```python
from build123d import *

# Parameters (mm, degrees)
ESTRUSIONE_ESTRUSIONE1_DEPTH = 5
SCHIZZO2_R                   = 1.625
TAGLIO_ESTRUSIONE1_DEPTH     = 11.10267083
SCHIZZO3_R                   = 2.5
TAGLIO_ESTRUSIONE2_DEPTH     = 3.5
RACCORDO1_R                  = 10
SCHIZZO4_W                   = 2.5
SCHIZZO4_H                   = 5
TAGLIO_ESTRUSIONE3_DEPTH     = 10
RACCORDO2_R                  = 1
SCHIZZO5_R                   = 1.625
TAGLIO_ESTRUSIONE4_DEPTH     = 10


with BuildPart() as part:
    # Schizzo1 → Estrusione-Estrusione1 (new body, symmetric)
    with BuildSketch(Plane(origin=(0, 0, 0), x_dir=(0, 0, -1), z_dir=(1, 0, 0))):
        Polygon((-21.188457268, 88.94490566), (-26.688457268, 88.94490566), (-26.688457268, 109.666731067), (-40, 122.978273799), (-40, 147.94490566), (-18, 169.94490566), (-16.585786438, 168.530692098), (-25, 160.116478536), (-25, 158.94490566), (-20, 158.94490566), (-34.5, 144.44490566), (-34.5, 125.256448392), (-21.188457268, 111.94490566), align=None)
    extrude(amount=ESTRUSIONE_ESTRUSIONE1_DEPTH, both=True)

    # Schizzo2 → Taglio-Estrusione1 (cut, through all)
    with BuildSketch(Plane.XY.offset(26.688457268)):
        with Locations((0, 92.723474812)):
            Circle(SCHIZZO2_R)
    extrude(amount=-TAGLIO_ESTRUSIONE1_DEPTH, mode=Mode.SUBTRACT)

    # Schizzo3 → Taglio-Estrusione2 (cut)
    with BuildSketch(Plane.XY.offset(26.688457268)):
        with Locations((0, 92.723474812)):
            Circle(SCHIZZO3_R)
    extrude(amount=-TAGLIO_ESTRUSIONE2_DEPTH, mode=Mode.SUBTRACT)

    # Raccordo1
    raccordo1_edges = [part.edges().sort_by_distance(p)[0] for p in [
        (0, 109.666731067, 26.688457268),
        (0, 122.978273799, 40),
        (0, 147.94490566, 40),
        (0, 144.44490566, 34.5),
        (0, 125.256448392, 34.5),
    ]]
    fillet(raccordo1_edges, radius=RACCORDO1_R)

    # Schizzo4 → Taglio-Estrusione3 (cut)
    with BuildSketch(Plane.ZY.offset(5)):
        with Locations((38.75, 141.44490566)):
            Rectangle(SCHIZZO4_W, SCHIZZO4_H)
    extrude(amount=-TAGLIO_ESTRUSIONE3_DEPTH, mode=Mode.SUBTRACT)

    # Raccordo2
    raccordo2_edges = [part.edges().sort_by_distance(p)[0] for p in [
        (0, 158.94490566, 25),
    ]]
    fillet(raccordo2_edges, radius=RACCORDO2_R)

    # Schizzo5 → Taglio-Estrusione4 (cut)
    with BuildSketch(Plane(origin=(0, 93.97245283, 93.97245283), x_dir=(1, 0, 0), z_dir=(0, 0.707106781, 0.707106781))):
        with Locations((0, 103.441273159)):
            Circle(SCHIZZO5_R)
    extrude(amount=-TAGLIO_ESTRUSIONE4_DEPTH, mode=Mode.SUBTRACT)


solid = part.part
```
Geometry check sheet. Reference: the model listing, model coordinates, mm. A direction names the side the tool comes from. Give positions to 0.01 mm unless a question says otherwise; leave off trailing zeros. Write each loop counter-clockwise with the first axis right and the second up, starting at its lowest first coordinate (ties: lowest second). Pieces come first, ordered by that corner, then holes.
1) Section check C-C, the plane x = 0. State how many separate pieces and enclosed holes the cut face has, and give its area (3 significant figures).
2) Section check B-B, the plane x = 4.25. Record the boundary of the cut face in (y, z).
3) Release check for a two-part mould opening along Z. For faces 4 (the flat face through (2, 93, 23.188)), 5 (the cylindrical face through (-0.07, 144.18, 33.718)), 6 (the cylindrical face through (-0.352, 165.298, 21.253)) record: pulls with the +Z half, pulls with the -Z half, needs draft (parallel to the pull), parting line crosses it, or undercut.
4) Section check A-A, the plane z = 28.5. Record the boundary of the cut face in (x, y), and give its area (3 significant figures).
5) Material ranges on L1, parallel to Y at x = 0, z = 25.85; L2, parallel to X at y = 93, z = 25.25; L3, parallel to Y at x = -1.5, z = 25.25, recorded low to high.
6) Section check D-D, the plane z = 33.5. Record the boundary of the cut face in (x, y), and give its area (3 significant figures).
7) Gauge pin test, flat ends, axial feed: pin 1 (1 mm diameter, centred on x = 2.5, y = 100.5, fed in from +Z); pin 2 (1.5 mm diameter, centred on x = -1, z = 29.5, fed in from -Y); pin 3 (3 mm diameter, centred on x = 0.5, z = 22, fed in from +Y). Record the tip position at first contact, or that the pin passes through.
8) Access from +Z, -Z, +X, -X, +Y, -Y to the whole of each face (thin tool, end or side, straight path). Record for faces 1 (the flat face through (0, 101, 21.188)), 2 (the flat face through (0, 138.945, 39)), 3 (the cylindrical face through (0.07, 125.521, 33.718)).
Computed:
1. separate pieces: 3
1. enclosed holes: 0
1. area: 449 mm2
2. outline: (88.94, 21.19) - (111.94, 21.19) - (122.33, 31.57) arc R10 cw to (129.4, 34.5) - (140.3, 34.5) arc R10 cw to (147.37, 31.57) - (158.94, 20) - (158.94, 24) arc R1 cw to (159.94, 25) - (160.12, 25) - (168.53, 16.59) - (169.94, 18) - (150.87, 37.07) arc R10 ccw to (143.94, 40) - (143.94, 37.5) - (138.94, 37.5) - (138.94, 40) - (127.12, 40) arc R10 ccw to (120.05, 37.07) - (112.6, 29.62) arc R10 cw to (105.52, 26.69) - (88.94, 26.69) - close
3. face 4: pulls with the +Z half
3. face 5: pulls with the -Z half
3. face 6: undercut
4. outline: (-5, 111.26) - (5, 111.26) - (5, 119.26) - (-5, 119.26) - close; (-5, 150.44) - (5, 150.44) - (5, 159.44) - (-5, 159.44) - close
4. area: 170 mm2
5. L1: y = 88.94 to 90.22, 95.22 to 116.61, 153.09 to 162.09
5. L2: x = -5 to -2.48, 2.48 to 5
5. L3: y = 88.94 to 90.72, 94.72 to 116.01, 153.69 to 162.69
6. outline: (-5, 116.48) - (5, 116.48) - (5, 125.04) - (-5, 125.04) - close; (-5, 144.66) - (5, 144.66) - (5, 154.44) - (-5, 154.44) - close
6. area: 183 mm2
7. pin 1: stops at z = 26.69
7. pin 2: stops at y = 111.61
7. pin 3: stops at y = 166.96
8. face 1: -Z, +X, -X, -Y
8. face 2: +Z, +X, -X
8. face 3: -Z, +X, -X
